```python
from build123d import *

# Parameters (mm, degrees)
BOSS_EXTRUDE1_DEPTH = 18.5
SKETCH3_R           = 8
BOSS_EXTRUDE2_DEPTH = 11
SKETCH4_R           = 2
BOSS_EXTRUDE3_DEPTH = 0.75
SKETCH6_R           = 1.5
BOSS_EXTRUDE4_DEPTH = 10
CUT_EXTRUDE1_DEPTH  = 10
CUT_EXTRUDE2_DEPTH  = 3


with BuildPart() as part:
    # Sketch2 → Boss-Extrude1 (new body)
    with BuildSketch(Plane(origin=(0, 0, 0), x_dir=(0, 0, -1), z_dir=(1, 0, 0))):
        with BuildLine():
            Line((0, 6), (-4.905354218, 6))
            ThreePointArc((-4.905354218, 6), (-7.75, 0), (-4.905354218, -6))
            Line((-4.905354218, -6), (0, -6))
            Line((0, -6), (0, 6))
        make_face()
        with BuildLine():
            Line((4.905354218, 6), (0, 6))
            Line((0, 6), (0, -6))
            Line((0, -6), (4.905354218, -6))
            ThreePointArc((4.905354218, -6), (7.002820688, -3.320090723), (7.75, 0))
            ThreePointArc((7.75, 0), (7.002820688, 3.320090723), (4.905354218, 6))
        make_face()
    extrude(amount=BOSS_EXTRUDE1_DEPTH)

    # Sketch3 → Boss-Extrude2 (add)
    with BuildSketch(Plane.ZY):
        Circle(SKETCH3_R)
    extrude(amount=BOSS_EXTRUDE2_DEPTH)

    # Sketch4 → Boss-Extrude3 (add)
    with BuildSketch(Plane.ZY.offset(11)):
        Circle(SKETCH4_R)
    extrude(amount=BOSS_EXTRUDE3_DEPTH)

    # Sketch6 → Boss-Extrude4 (add)
    with BuildSketch(Plane.ZY.offset(11.75)):
        Circle(SKETCH6_R)
    extrude(amount=BOSS_EXTRUDE4_DEPTH)

    # Sketch7 → Cut-Extrude1 (cut)
    with BuildSketch(Plane.ZY.offset(21.75)):
        Polygon((-36.741347109, 1), (-1.118033989, 1), (1.118033989, 1), (36.741347109, 1), (36.741347109, 72.246626241), (-36.741347109, 72.246626241), align=None)
    extrude(amount=-CUT_EXTRUDE1_DEPTH, mode=Mode.SUBTRACT)

    # Sketch8 → Cut-Extrude2 (cut)
    with BuildSketch(Plane.ZY.offset(11)):
        with BuildLine():
            ThreePointArc((-4.388888889, -0.99380799), (-3.754644008, -0.666666667), (-3.5, 0))
            Line((-3.5, 0), (-4.5, 0))
            ThreePointArc((-4.5, 0), (-4.472135955, -0.5), (-4.388888889, -0.99380799))
        make_face()
        with BuildLine():
            Line((-4.5, 0), (-3.5, 0))
            ThreePointArc((-3.5, 0), (-3.754644008, 0.666666667), (-4.388888889, 0.99380799))
            ThreePointArc((-4.388888889, 0.99380799), (-4.472135955, 0.5), (-4.5, 0))
        make_face()
        with BuildLine():
            ThreePointArc((-4.5, 0), (-4.472135955, 0.5), (-4.388888889, 0.99380799))
            ThreePointArc((-4.388888889, 0.99380799), (-5.166666667, 0.745355992), (-5.5, 0))
            Line((-5.5, 0), (-4.5, 0))
        make_face()
        with BuildLine():
            ThreePointArc((-5.5, 0), (-5.166666667, -0.745355992), (-4.388888889, -0.99380799))
            ThreePointArc((-4.388888889, -0.99380799), (-4.472135955, -0.5), (-4.5, 0))
            Line((-4.5, 0), (-5.5, 0))
        make_face()
        with BuildLine():
            ThreePointArc((4.388888889, 0.99380799), (4.472135955, 0.5), (4.5, 0))
            Line((4.5, 0), (5.5, 0))
            ThreePointArc((5.5, 0), (5.166666667, 0.745355992), (4.388888889, 0.99380799))
        make_face()
        with BuildLine():
            ThreePointArc((4.388888889, -0.99380799), (4.472135955, -0.5), (4.5, 0))
            Line((4.5, 0), (3.5, 0))
            ThreePointArc((3.5, 0), (3.754644008, -0.666666667), (4.388888889, -0.99380799))
        make_face()
        with BuildLine():
            Line((3.5, 0), (4.5, 0))
            ThreePointArc((4.5, 0), (4.472135955, 0.5), (4.388888889, 0.99380799))
            ThreePointArc((4.388888889, 0.99380799), (3.754644008, 0.666666667), (3.5, 0))
        make_face()
        with BuildLine():
            Line((5.5, 0), (4.5, 0))
            ThreePointArc((4.5, 0), (4.472135955, -0.5), (4.388888889, -0.99380799))
            ThreePointArc((4.388888889, -0.99380799), (5.166666667, -0.745355992), (5.5, 0))
        make_face()
    extrude(amount=-CUT_EXTRUDE2_DEPTH, mode=Mode.SUBTRACT)


solid = part.part
```
For this review, take the finished solid that the model builds, in its own axes (mm). A direction names the side the tool comes from. Round coordinates to 2 decimals unless told otherwise and drop trailing zeros. Order: outer loops, then holes, each group sorted by start corner. A loop starts at its lowest first (then second) coordinate and runs counter-clockwise, first axis right, second up. Notation, with made-up numbers: (58, -12.75) -> (97, -12.75) arc R11 cw to (97, -6.75) -> close; hole circle Ø8 at (19.5, -36.75). An arc over 180 degrees is marked (long way). Use a Markdown table: item, result.
Item 1: For line 1 along X through (y, z) = (-7.5, 1.5); line 2 along X through (y, z) = (-1.75, -7); line 3 along Y through (x, z) = (7, 6), list the stretches that pass through material, from the lowest coordinate up. Write a range as [from, to].
Resolved:
| item | result |
|---|---|
| line 1 | x = [-11, 0] |
| line 2 | x = [-11, 18.5] |
| line 3 | y = [-4.91, 4.91] |
Item 2: Take a section at D-D (y = -5). State the section outline as (x, z) points (3 decimals), plus the area to 3 significant figures.
Resolved:
| item | result |
|---|---|
| outline | (-11, -6.245) -> (0, -6.245) -> (0, -5.921) -> (18.5, -5.921) -> (18.5, 5.921) -> (0, 5.921) -> (0, 6.245) -> (-11, 6.245) -> close |
| area | 356 mm² |
Item 3: Take a section at C-C (x = 8). State the section outline as (y, z) points.
Resolved:
| item | result |
|---|---|
| outline | (-6, -4.91) arc R7.75 ccw to (6, -4.91) -> (6, 4.91) arc R7.75 ccw to (-6, 4.91) -> close |
Item 4: For pin 1 (5 mm diameter, centred on y = 4, z = 3.5, fed in from -X); pin 2 (1.5 mm diameter, centred on x = 3, y = 4.5, fed in from -Z); pin 3 (3 mm diameter, centred on x = 13, z = 1, fed in from +Y), all flat-tipped, find the tip position at first contact; note any pin that passes through.
Resolved:
| item | result |
|---|---|
| pin 1 | stops at x = -11 |
| pin 2 | stops at z = -6.78 |
| pin 3 | stops at y = 6 |
Item 5: Draft analysis for pull direction Z (two halves, no side actions). For faces 5 (the cylindrical face through (-16.7, -1.5, 0)), 6 (the flat face through (-17, 1, 0)), 7 (the flat face through (-8, 0, -5)), state which applies: +Z half, -Z half, draft (parallel to the pull), parting line (faces both ways), or undercut.
Resolved:
| item | result |
|---|---|
| face 5 | parting line |
| face 6 | draft |
| face 7 | undercut |
Item 6: Machinability: for faces 1 (the flat face through (9, -6, 0)), 2 (the cylindrical face through (9.12, 0.1, 7.75)), 3 (the cylindrical face through (-11.37, -1.952, -0.434)), 4 (the flat face through (9, 6, 0)), which of the approach directions +Z, -Z, +X, -X, +Y, -Y give a long, thin tool a straight path to every point of the face, cutting with its end or side? Answer none if there is none.
Resolved:
| item | result |
|---|---|
| face 1 | +Z, -Z, +X, -Y |
| face 2 | +Z, +X |
| face 3 | -X |
| face 4 | +Z, -Z, +X, +Y |
Item 7: Take a section at B-B (y = -2.5). State the section outline as (x, z) points.
Resolved:
| item | result |
|---|---|
| outline | (-11, -7.6) -> (0, -7.6) -> (0, -7.34) -> (18.5, -7.34) -> (18.5, 7.34) -> (0, 7.34) -> (0, 7.6) -> (-11, 7.6) -> close |
Item 8: Take a section at A-A (z = 0). State the section outline as (x, y) points.
Resolved:
| item | result |
|---|---|
| outline | (-21.75, -1.5) -> (-11.75, -1.5) -> (-11.75, -2) -> (-11, -2) -> (-11, -8) -> (0, -8) -> (0, -6) -> (18.5, -6) -> (18.5, 6) -> (0, 6) -> (0, 8) -> (-11, 8) -> (-11, 2) -> (-11.75, 2) -> (-11.75, 1) -> (-21.75, 1) -> close |
